Part model, mm, in its own coordinate system. A direction names the side the tool comes from. Round coordinates to 2 decimals unless told otherwise and drop trailing zeros. Write each loop counter-clockwise with the first axis right and the second up, starting at its lowest first coordinate (ties: lowest second). Pieces come first, ordered by that corner, then holes.
1) Pull direction Y, two halves, no side cores. Call faces 1 (the cylindrical face through (44.539, 36.185, -23.608)), 2 (the flat face through (-15, 66.35, 5)), 3 (the cylindrical face through (44.539, 33.664, -2.247)), 4 (the cylindrical face through (22.665, 68.124, -2.976)): +Y half, -Y half, draft (parallel to the pull), parting line (faces both ways), or undercut.
2) Drill centre lines: L1, parallel to Z at x = 45, y = 38; L2, parallel to X at y = 5, z = 33. Where is each one in solid material? Low to high.
3) Saw through at D-D on z = 0. Write the cut outline in (x, y), and give its area (3 significant figures).
4) Saw through at B-B on x = 0. Write the cut outline in (y, z), and give its area (3 significant figures).
5) Flat gauge pins, fed straight in: pin 1 (1.5 mm diameter, centred on x = 4, z = 28, fed in from -Y); pin 2 (8 mm diameter, centred on y = 38.1, z = -18.99, fed in from +X); pin 3 (23 mm diameter, centred on x = 9.5, z = 4.5, fed in from +Y). Where does each tip first touch, or does it go through?
6) Which spindle directions (+Z, -Z, +X, -X, +Y, -Y) get a long thin tool onto all of the face, cutting with end or side? Do faces 5 (the flat face through (38.1, 73, 1)), 6 (the flat face through (50.8, 46, 1)), 7 (the flat face through (16, 64.85, -1)). Say none if no direction does.
7) Saw through at C-C on y = 15.5. Write the cut outline in (x, z), and give its area (3 significant figures).
8) Saw through at A-A on y = 38.1. Write the cut outline in (x, z).
```python
from build123d import *

# Parameters (mm, degrees)
SKETCH1_W           = 101.6
SKETCH1_H           = 101.6
SKETCH1_W_2         = 76.2
SKETCH1_H_2         = 76.2
BOSS_EXTRUDE1_DEPTH = 76.2
BOSS_EXTRUDE2_START = -6.35
SKETCH2_W           = 76.2
SKETCH2_H           = 76.2
SKETCH2_R           = 15.24
BOSS_EXTRUDE2_DEPTH = 5
SKETCH3_R           = 22.86
CUT_EXTRUDE2_DEPTH  = 3.5
SKETCH4_R           = 5
CUT_EXTRUDE3_DEPTH  = 12.7


with BuildPart() as part:
    # Sketch1 → Boss-Extrude1 (new body)
    with BuildSketch(Plane(origin=(0, 0, 0), x_dir=(1, 0, 0), z_dir=(0, 1, 0))):
        Rectangle(SKETCH1_W, SKETCH1_H)
        Rectangle(SKETCH1_W_2, SKETCH1_H_2, mode=Mode.SUBTRACT)
    extrude(amount=BOSS_EXTRUDE1_DEPTH)

    # Sketch2 → Boss-Extrude2 (add)
    with BuildSketch(Plane(origin=(0, 76.2, 0), x_dir=(1, 0, 0), z_dir=(0, 1, 0)).offset(BOSS_EXTRUDE2_START)):
        Rectangle(SKETCH2_W, SKETCH2_H)
        with Locations(Location((0, 0, 0), (0, 0, 270))):
            Circle(SKETCH2_R, mode=Mode.SUBTRACT)
    extrude(amount=-BOSS_EXTRUDE2_DEPTH)

    # Sketch3 → Cut-Extrude2 (cut)
    with BuildSketch(Plane(origin=(0, 69.85, 0), x_dir=(1, 0, 0), z_dir=(0, 1, 0))):
        with Locations(Location((0, 0, 0), (0, 0, 270))):
            Circle(SKETCH3_R)
    extrude(amount=-CUT_EXTRUDE2_DEPTH, mode=Mode.SUBTRACT)

    # Sketch4 → Cut-Extrude3 (cut)
    with BuildSketch(Plane(origin=(50.8, 0, 0), x_dir=(0, 0, -1), z_dir=(1, 0, 0))):
        with Locations((-19.110683009, 38.1)):
            Circle(SKETCH4_R)
        with Locations((-0.060683009, 38.1)):
            Circle(SKETCH4_R)
        with Locations((18.989316991, 38.1)):
            Circle(SKETCH4_R)
    extrude(amount=-CUT_EXTRUDE3_DEPTH, mode=Mode.SUBTRACT)


solid = part.part
```
Completed:
1. face 1: undercut
1. face 2: +Y half
1. face 3: undercut
1. face 4: draft
2. L1: z = -50.8 to -23.99, -13.99 to -4.94, 5.06 to 14.11, 24.11 to 50.8
2. L2: x = -50.8 to -38.1, 38.1 to 50.8
3. outline: (-50.8, 0) - (-38.1, 0) - (-38.1, 64.85) - (-15.24, 64.85) - (-15.24, 66.35) - (-22.86, 66.35) - (-22.86, 69.85) - (-38.1, 69.85) - (-38.1, 76.2) - (-50.8, 76.2) - close; (15.24, 64.85) - (38.1, 64.85) - (38.1, 43.1) - (50.8, 43.1) - (50.8, 76.2) - (38.1, 76.2) - (38.1, 69.85) - (22.86, 69.85) - (22.86, 66.35) - (15.24, 66.35) - close; (38.1, 0) - (50.8, 0) - (50.8, 33.1) - (38.1, 33.1) - close
3. area: 1,980 mm2
4. outline: (0, -50.8) - (76.2, -50.8) - (76.2, -38.1) - (69.85, -38.1) - (69.85, -22.86) - (66.35, -22.86) - (66.35, -15.24) - (64.85, -15.24) - (64.85, -38.1) - (0, -38.1) - close; (0, 38.1) - (64.85, 38.1) - (64.85, 15.24) - (66.35, 15.24) - (66.35, 22.86) - (69.85, 22.86) - (69.85, 38.1) - (76.2, 38.1) - (76.2, 50.8) - (0, 50.8) - close
4. area: 2,110 mm2
5. pin 1: stops at y = 64.85
5. pin 2: stops at x = -38.1
5. pin 3: stops at y = 66.35
6. face 5: +Y
6. face 6: +Z, -Z, +X, +Y, -Y
6. face 7: -Y
7. outline: (-50.8, -50.8) - (50.8, -50.8) - (50.8, 50.8) - (-50.8, 50.8) - close; hole (-38.1, -38.1) - (38.1, -38.1) - (38.1, 38.1) - (-38.1, 38.1) - close
7. area: 4,520 mm2
8. outline: (-50.8, -50.8) - (50.8, -50.8) - (50.8, -23.99) - (38.1, -23.99) - (38.1, -38.1) - (-38.1, -38.1) - (-38.1, 38.1) - (38.1, 38.1) - (38.1, 24.11) - (50.8, 24.11) - (50.8, 50.8) - (-50.8, 50.8) - close; (38.1, -13.99) - (50.8, -13.99) - (50.8, -4.94) - (38.1, -4.94) - close; (38.1, 5.06) - (50.8, 5.06) - (50.8, 14.11) - (38.1, 14.11) - close
